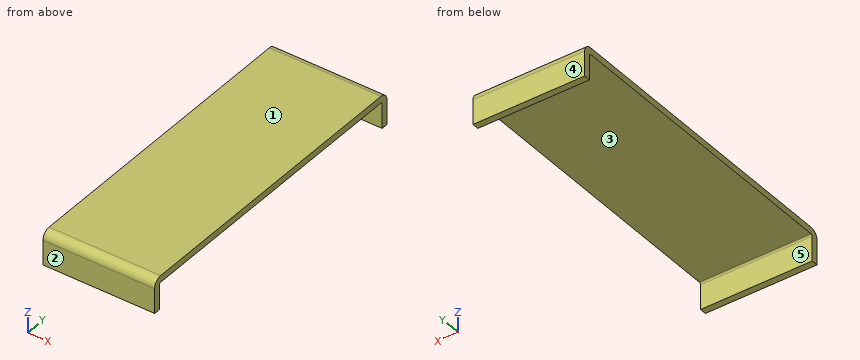
```python
from build123d import *

# Parameters (mm, degrees)
SKETCH1_W                    = 50.580870405
SKETCH1_H                    = 144
BASE_FLANGE1_DEPTH           = 3
EDGE_FLANGE1_STRIP_W         = 13.4732
EDGE_FLANGE1_STRIP_H         = 3
EDGE_FLANGE1_STRIP_CUT_DEPTH = 50.580870405
EDGE_FLANGE1_DEPTH           = 50.580870405
EDGE_FLANGE2_STRIP_W         = 13.4732
EDGE_FLANGE2_STRIP_H         = 3
EDGE_FLANGE2_STRIP_CUT_DEPTH = 50.580870405
EDGE_FLANGE2_DEPTH           = 50.580870405


# Sheet-metal steps are written as plain solids
with BuildPart() as part:
    # Sketch1 → Base-Flange1 (new body)
    with BuildSketch(Plane.XY):
        with Locations((46.586592155, 25.88784612)):
            Rectangle(SKETCH1_W, SKETCH1_H)
    extrude(amount=-BASE_FLANGE1_DEPTH)

    # Edge-Flange1 strip (across the edge) → Edge-Flange1 strip cut (cut)
    with BuildSketch(Plane(origin=(71.877027357, -46.11215388, -3), x_dir=(0, 1, 0), z_dir=(-1, 0, 0))):
        with Locations((-3, -1.5)):
            Rectangle(EDGE_FLANGE1_STRIP_W, EDGE_FLANGE1_STRIP_H)
    extrude(amount=EDGE_FLANGE1_STRIP_CUT_DEPTH, mode=Mode.SUBTRACT)

    # Edge-Flange1 section (across the edge) → Edge-Flange1 (add)
    with BuildSketch(Plane(origin=(71.877027357, -46.11215388, -3), x_dir=(0, 1, 0), z_dir=(-1, 0, 0))):
        with BuildLine():
            Line((0, 0.7366), (0, 12))
            Line((0, 12), (3, 12))
            Line((3, 12), (3, 0.7366))
            ThreePointArc((3, 0.7366), (3.215745145, 0.215745145), (3.7366, 0))
            Line((3.7366, 0), (3.7366, -3))
            ThreePointArc((3.7366, -3), (1.094424801, -1.905575199), (0, 0.7366))
        make_face()
    extrude(amount=EDGE_FLANGE1_DEPTH)

    # Edge-Flange2 strip (across the edge) → Edge-Flange2 strip cut (cut)
    with BuildSketch(Plane(origin=(21.296156952, 97.88784612, -3), x_dir=(0, -1, 0), z_dir=(1, 0, 0))):
        with Locations((-3, -1.5)):
            Rectangle(EDGE_FLANGE2_STRIP_W, EDGE_FLANGE2_STRIP_H)
    extrude(amount=EDGE_FLANGE2_STRIP_CUT_DEPTH, mode=Mode.SUBTRACT)

    # Edge-Flange2 section (across the edge) → Edge-Flange2 (add)
    with BuildSketch(Plane(origin=(21.296156952, 97.88784612, -3), x_dir=(0, -1, 0), z_dir=(1, 0, 0))):
        with BuildLine():
            Line((0, 0.7366), (0, 12))
            Line((0, 12), (3, 12))
            Line((3, 12), (3, 0.7366))
            ThreePointArc((3, 0.7366), (3.215745145, 0.215745145), (3.7366, 0))
            Line((3.7366, 0), (3.7366, -3))
            ThreePointArc((3.7366, -3), (1.094424801, -1.905575199), (0, 0.7366))
        make_face()
    extrude(amount=EDGE_FLANGE2_DEPTH)


solid = part.part
```
Part model, mm, in its own coordinate system. Face numbers are marked on the shaded views. A direction names the side the tool comes from. Coordinates: 2 decimals unless noted, no trailing zeros. Loops run counter-clockwise (first coordinate to the right, second up) from the corner with the lowest first, then second, coordinate; pieces in that order, holes last. Notation, with made-up numbers: (-34, -27) - (-16, -27) arc R15 cw to (-16, -20) - close; hole circle Ø5 at (-13.5, 86). An arc over 180 degrees is marked (long way). Write item = value, one per line. Start each with the question number.
Item 1: Mould opens along Y. For the marked faces 1, 2 and 3 say: released by +Y, released by -Y, zero draft, split by the parting line, or undercut.
Item 2: Cut at A-A, the plane z = -10.5. Give the cut face in (x, y), and give its area (3 significant figures).
Item 3: Cut at C-C, the plane y = 30. Give the cut face in (x, z), and give its area (3 significant figures).
Item 4: 3-axis set-ups, long thin cutter, end or side, ignore diameter. For the marked faces 4 and 5: which of +Z, -Z, +X, -X, +Y, -Y reach the whole face in a straight line?
Item 5: Flat gauge pin, fed straight in: pin 1 Ø4 at (x, y) = (37, 71.5) entering from -Z. Where does the tip first touch, or does it go through?
Item 6: Cut at B-B, the plane x = 46. Give the cut face in (y, z).
Item 7: Wall check: L1, parallel to Y at x = 48.5, z = -7.5; L2, parallel to Z at x = 64, y = 24.5; L3, parallel to Y at x = 67.5, z = -0.75. Give the ranges that are in metal, low to high. Write a range as from..to.
The answers:
q1.face_1 = zero draft
q1.face_2 = released by -Y
q1.face_3 = undercut
q2.outline = (21.3, -46.11) - (71.88, -46.11) - (71.88, -43.11) - (21.3, -43.11) - close; (21.3, 94.89) - (71.88, 94.89) - (71.88, 97.89) - (21.3, 97.89) - close
q2.area = 303 mm2
q3.outline = (21.3, -3) - (71.88, -3) - (71.88, 0) - (21.3, 0) - close
q3.area = 152 mm2
q4.face_4 = +Z, -Z, +X, -X, +Y
q4.face_5 = -Z, +X, -X
q5.pin_1 = -3
q6.outline = (-46.11, -15) - (-43.11, -15) - (-43.11, -3.74) arc R0.74 cw to (-42.38, -3) - (94.15, -3) arc R0.74 cw to (94.89, -3.74) - (94.89, -15) - (97.89, -15) - (97.89, -3.74) arc R3.74 ccw to (94.15, 0) - (-42.38, 0) arc R3.74 ccw to (-46.11, -3.74) - close
q7.L1 = -46.11..-43.11, 94.89..97.89
q7.L2 = -3..0
q7.L3 = -44.62..96.4
